Geometry check sheet. Reference: the model listing, model coordinates, mm. A direction names the side the tool comes from. Round coordinates to 2 decimals unless told otherwise and drop trailing zeros. Order: outer loops, then holes, each group sorted by start corner. A loop starts at its lowest first (then second) coordinate and runs counter-clockwise, first axis right, second up. Notation, with made-up numbers: (-0.75, 49) - (40.25, 49) arc R16 ccw to (40.25, 65) - close; hole circle Ø6 at (-8.5, -35). An arc over 180 degrees is marked (long way). One line per question, with ' | ' between items. Start each with the question number.
Q1. Sectioned sample at D-D, the plane y = 0. Enter the section's corners in (x, z).
Q2. Sectioned sample at A-A, the plane z = 5. Enter the section's corners in (x, y), then the cut area to 3 significant figures.
Q3. Mould release check, pull along Y, two halves, no side actions. Record for faces 1 (the face through (-0.2, -42.2, 6.4)), 2 (the face through (2, -10, -4.013)), 3 (the face through (-0.94, 41.27, -0.03)), 4 (the face through (0, -51.5, 0)): +Y half, -Y half, draft (parallel to the pull), parting line (faces both ways), or undercut.
Q4. Sectioned sample at C-C, the plane x = 8.5. Enter the section's corners in (y, z).
Q5. Material ranges on line 1 along X through (y, z) = (-39, 0.5); line 2 along Y through (x, z) = (10.75, 3.75); line 3 along Y through (x, z) = (-1.75, 4.75), recorded low to high.
Q6. Tool access check on faces 5 (the face through (0, 28.05, 3)), 6 (the face through (-7, -3.4, -4.013)), 7 (the face through (-12.7, -1, -1)). Record the directions out of +Z, -Z, +X, -X, +Y, -Y that give a thin tool (end or side, any length) a straight path to the whole face; none if there is none.
Q7. Sectioned sample at B-B, the plane y = -39. Enter the section's corners in (x, z), then the cut area to 3 significant figures.
Q8. Gauge pin test, flat ends, axial feed: P1, Ø1.5, axis at x = 6.5, y = 2.5, coming from the +Z side; P2, Ø11.5, axis at x = -9.5, y = 0, coming from the +Z side. Record the tip position at first contact, or that the pin passes through.
Autodesk Inventor part; units mm, degrees
ref_plane "screw1_XY" through (-6.905, 0, -4.0132) normal (0, 0, 1) x (1, 0, 0)
ref_plane "screw1_YZ" through (-6.905, 0, -4.0132) normal (1, 0, 0) x (0, 1, 0)
ref_plane "screw1_ZX" through (-6.905, 0, -4.0132) normal (0, 1, 0) x (0, 0, 1)
sketch "Sketch_1" plane through (0, 0, 0) normal (1, 0, 0) x (0, 1, 0)
  line L0 (-28.05, 6.4) -> (-51.5, 6.4)
  line L1 (-51.5, 6.4) -> (-51.5, -6.3)
  line L2 (-51.5, -6.3) -> (51.5, -6.3)
  line L3 (51.5, -6.3) -> (51.5, 6.4)
  line L4 (51.5, 6.4) -> (28.05, 6.4)
  line L5 (28.05, 6.4) -> (28.05, 0)
  line L6 (28.05, 0) -> (-28.05, 0)
  line L7 (-28.05, 0) -> (-28.05, 6.4)
extrude "Extrusion1" add sketch "Sketch_1" along normal mid plane 25.4
sketch "Sketch_2" plane through (0, 0, 0) normal (1, 0, 0) x (0, 1, 0)
  line L0 (39, -6.3) -> (39, 6.4)
  line L1 (39, 6.4) -> (42, 6.4)
  line L2 (42, 6.4) -> (41.4585, 5.8585)
  line L3 (41.4585, 5.8585) -> (41.4585, -5.7585)
  line L4 (41.4585, -5.7585) -> (42, -6.3)
  line L5 (42, -6.3) -> (39, -6.3)
  line L6 (39, -6.3) -> (39, 6.4)
revolve "Revolution1" cut sketch "Sketch_2" angle 360 about axis through (0, 39, -6.3) along (0, 0, -1)
thread "Thread1"
sketch "Sketch_3" plane through (0, 0, 0) normal (1, 0, 0) x (0, 1, 0)
  line L0 (-39, -6.3) -> (-39, 6.4)
  line L1 (-39, 6.4) -> (-36, 6.4)
  line L2 (-36, 6.4) -> (-36.5415, 5.8585)
  line L3 (-36.5415, 5.8585) -> (-36.5415, -5.7585)
  line L4 (-36.5415, -5.7585) -> (-36, -6.3)
  line L5 (-36, -6.3) -> (-39, -6.3)
  line L6 (-39, -6.3) -> (-39, 6.4)
revolve "Revolution2" cut sketch "Sketch_3" angle 360 about axis through (0, -39, -6.3) along (0, 0, -1)
thread "Thread2"
sketch "Sketch4" plane through (-12.7, -28.05, 0) normal (0, 0, 1) x (1, 0, 0)
  point P0 (5.795, 28.05)
hole "Hole1" at (-6.905, 0, 0) direction (0, 0, -1) diameter 6.2992 depth 6.3 counterbore diameter 10.3124 counterbore depth 4.0132
pattern_linear "Rectangular Pattern1" count 2 spacing 14.4558 along (0.4777, 0.8785, 0) count 2 spacing 14.4558 along (0.4777, -0.8785, 0) of "Hole1"
ref_plane "screw1_XY" through (-6.905, 0, -4.0132) normal (0, 0, 1) x (1, 0, 0)
ref_plane "screw1_YZ" through (-6.905, 0, -4.0132) normal (1, 0, 0) x (0, 1, 0)
ref_plane "screw1_ZX" through (-6.905, 0, -4.0132) normal (0, 1, 0) x (0, 0, 1)
ref_plane "screw1_1_XY" through (0, 12.7, -4.0132) normal (0, 0, 1) x (1, 0, 0)
ref_plane "screw1_1_YZ" through (0, 12.7, -4.0132) normal (1, 0, 0) x (0, 1, 0)
ref_plane "screw1_1_ZX" through (0, 12.7, -4.0132) normal (0, 1, 0) x (0, 0, 1)
ref_plane "screw2_XY" through (6.905, 0, -4.0132) normal (0, 0, 1) x (1, 0, 0)
ref_plane "screw2_YZ" through (6.905, 0, -4.0132) normal (1, 0, 0) x (0, 1, 0)
ref_plane "screw2_ZX" through (6.905, 0, -4.0132) normal (0, 1, 0) x (0, 0, 1)
ref_plane "screw2_1_XY" through (0, -12.7, -4.0132) normal (0, 0, 1) x (1, 0, 0)
ref_plane "screw2_1_YZ" through (0, -12.7, -4.0132) normal (1, 0, 0) x (0, 1, 0)
ref_plane "screw2_1_ZX" through (0, -12.7, -4.0132) normal (0, 1, 0) x (0, 0, 1)
ref_plane "to_dummy_XY" through (0, 0, 0) normal (0, 0, 1) x (1, 0, 0)
ref_plane "to_dummy_YZ" through (0, 0, 0) normal (1, 0, 0) x (0, 1, 0)
ref_plane "to_dummy_ZX" through (0, 0, 0) normal (0, 1, 0) x (0, 0, 1)
ref_plane "to_wheel1_XY" through (0, 39, 6.4) normal (0, 0, 1) x (1, 0, 0)
ref_plane "to_wheel1_YZ" through (0, 39, 6.4) normal (1, 0, 0) x (0, 1, 0)
ref_plane "to_wheel1_ZX" through (0, 39, 6.4) normal (0, 1, 0) x (0, 0, 1)
ref_plane "to_wheel2_XY" through (0, -39, 6.4) normal (0, 0, 1) x (1, 0, 0)
ref_plane "to_wheel2_YZ" through (0, -39, 6.4) normal (1, 0, 0) x (0, 1, 0)
ref_plane "to_wheel2_ZX" through (0, -39, 6.4) normal (0, 1, 0) x (0, 0, 1)
sketch "Sketch5" plane through (12.7, 0, 0) normal (1, 0, 0) x (0, 0, -1)
  line L0 (-5.8585, 36.5415) -> (-5.8585, 41.4585)
  line L1 (-5.8585, 39) -> (-5.8585, -3)
  line L2 (-6.4, 28.05) -> (0, 28.05)
  line L3 (6.3, -51.5) -> (6.3, 51.5)
  line L4 (-6.4, 28.05) -> (6.3, 28.05)
  line L5 (6.3, 28.05) -> (6.3, -51.5)
  line L6 (6.3, -51.5) -> (-6.4, -51.5)
  line L7 (-6.4, -51.5) -> (-6.4, 28.05)
  point P0 (0, 0)
  dimension "d28" = 42
properties part number "25-2752-1_p"
Determined:
1) outline: (-12.7, -6.3) - (-10.05, -6.3) - (-10.05, -4.01) - (-12.06, -4.01) - (-12.06, 0) - (-12.7, 0) - close; (-3.76, -6.3) - (3.76, -6.3) - (3.76, -4.01) - (1.75, -4.01) - (1.75, 0) - (-1.75, 0) - (-1.75, -4.01) - (-3.76, -4.01) - close; (10.06, -6.3) - (12.7, -6.3) - (12.7, 0) - (12.06, 0) - (12.06, -4.01) - (10.06, -4.01) - close
2) outline: (-12.7, -51.5) - (12.7, -51.5) - (12.7, -28.05) - (-12.7, -28.05) - close; (-12.7, 28.05) - (12.7, 28.05) - (12.7, 51.5) - (-12.7, 51.5) - close; hole circle Ø4.92 at (0, -39); hole circle Ø4.92 at (0, 39) | area: 1,150 mm2
3) face 1: draft | face 2: undercut | face 3: undercut | face 4: -Y half
4) outline: (-51.5, -6.3) - (-2.72, -6.3) - (-2.72, -4.01) - (-4.9, -4.01) - (-4.9, 0) - (-28.05, 0) - (-28.05, 6.4) - (-51.5, 6.4) - close; (2.72, -6.3) - (51.5, -6.3) - (51.5, 6.4) - (28.05, 6.4) - (28.05, 0) - (4.9, 0) - (4.9, -4.01) - (2.72, -4.01) - close
5) line 1: x = -12.7 to -2.46, 2.46 to 12.7 | line 2: y = -51.5 to -28.05, 28.05 to 51.5 | line 3: y = -51.5 to -40.73, -37.27 to -28.05, 28.05 to 37.27, 40.73 to 51.5
6) face 5: +Z, +X, -X | face 6: +Z | face 7: +Z, -Z, -X, +Y, -Y
7) outline: (-12.7, -6.3) - (-3, -6.3) - (-2.46, -5.76) - (-2.46, 5.86) - (-3, 6.4) - (-12.7, 6.4) - close; (2.46, -5.76) - (3, -6.3) - (12.7, -6.3) - (12.7, 6.4) - (3, 6.4) - (2.46, 5.86) - close | area: 260 mm2
8) P1: stops at z = -4.01 | P2: stops at z = 0
